Geometry check sheet. Reference: the model listing, model coordinates, mm. Round coordinates to 2 decimals unless told otherwise and drop trailing zeros. Order: outer loops, then holes, each group sorted by start corner. A loop starts at its lowest first (then second) coordinate and runs counter-clockwise, first axis right, second up.
(1) Cross-section at B-B on y = 24.5. Enter the section's corners in (x, z).
(2) Thickness scan on L1, parallel to Y at x = 1.8, z = -2.15; L2, parallel to X at y = -25, z = 1.25; L3, parallel to X at y = -37, z = -1.75. Record the ranges inside material, lowest first.
(3) Gauge pin test, flat ends, axial feed: P1, Ø10, axis at x = -2, y = 32.5, coming from the +Z side; P2, Ø4.5, axis at x = -55, y = 36, coming from the +Z side; P3, Ø2.5, axis at y = 6.5, z = -2, coming from the -X side; P4, Ø1.7, axis at x = 60, y = -36.5, coming from the +Z side. Record the tip position at first contact, or that the pin passes through.
(4) Cross-section at A-A on x = 50.1. Enter the section's corners in (y, z).
(5) Cross-section at C-C on x = 15. Enter the section's corners in (y, z), and give its area (3 significant figures).
Autodesk Inventor part; units mm, degrees
ref_plane "YZ Plane" through (0, 0, 0) normal (1, 0, 0) x (0, 1, 0)
ref_plane "XZ Plane" through (0, 0, 0) normal (0, 1, 0) x (-1, 0, 0)
ref_plane "XY Plane" through (0, 0, 0) normal (0, 0, 1) x (1, 0, 0)
sketch "Sketch1" plane through (0, 0, 0) normal (0, 0, 1) x (1, 0, 0)
  line L0 (65, -35) -> (-65, -35)
  line L1 (-65, -35) -> (-65, 35)
  line L2 (-65, 35) -> (65, 35)
  line L3 (65, 35) -> (65, -35)
  line L4 (65, -35) -> (-65, 35) construction
  line L5 (-65, -35) -> (65, 35) construction
  line L6 (56.8, -15) -> (56.8, -25) construction
  line L7 (54.65, -15) -> (54.65, -25)
  line L8 (58.95, -25) -> (58.95, -15)
  arc A0 (58.95, -15) -> (54.65, -15) centre (56.8, -15) ccw
  arc A1 (54.65, -25) -> (58.95, -25) centre (56.8, -25) ccw
  line L9 (62, -13) -> (65, -13)
  line L10 (65, -13) -> (65, -27)
  line L11 (65, -27) -> (62, -27)
  line L12 (62, -27) -> (62, -13)
  line L13 (62, -13) -> (65, -27) construction
  line L14 (65, -13) -> (62, -27) construction
  line L15 (56.8, -20) -> (63.5, -20) construction
  line L16 (48.6, -13) -> (51.6, -13)
  line L17 (51.6, -13) -> (51.6, -27)
  line L18 (51.6, -27) -> (48.6, -27)
  line L19 (48.6, -27) -> (48.6, -13)
  line L20 (48.6, -13) -> (51.6, -27) construction
  line L21 (51.6, -13) -> (48.6, -27) construction
  line L22 (50.1, -20) -> (56.8, -20) construction
  circle A2 centre (56.8, -20) radius 0.5
  line L23 (56.8, -20) -> (-65, -20)
  line L24 (-60, 35) -> (-60, -35)
  line L25 (-65, 35) -> (65, 35)
  line L26 (65, 35) -> (65, 41)
  line L27 (65, 41) -> (-65, 41)
  line L28 (-65, 41) -> (-65, 35)
  line L29 (-60, 35) -> (-60, 41)
  circle A3 centre (50.1, -13) radius 1.5
  circle A4 centre (63.5, -13) radius 1.5
  circle A5 centre (50.1, -27) radius 1.5
  circle A6 centre (63.5, -27) radius 1.5
  line L30 (-65, -35) -> (-65, -41)
  line L31 (-65, -41) -> (65, -41)
  line L32 (65, -41) -> (65, -35)
  line L33 (-60, -35) -> (-60, -41)
  point P0 (0, 0)
  point P1 (65, -27)
  point P2 (65, -13)
  point P3 (65, -13)
  dimension "d0" = 70
  dimension "d1" = 130
  dimension "d2" = 10
  dimension "d3" = 4.3
  dimension "d4" = 14
  dimension "d5" = 3
  dimension "d6" = 14
  dimension "d7" = 3
  dimension "d10" = 8
  dimension "d11" = 0
  dimension "d16" = 1
  dimension "d20" = 5.2
  dimension "d21" = 5.2
  dimension "d22" = 5
  dimension "d23" = 6
  dimension "d26" = 125
  dimension "d27" = 76
  dimension "d122" = 6
extrude "Extrusion1" add sketch "Sketch1" against normal blind 5 contours L32 L31 L33 L0 | L19 A3 L17 L23 | L23 L17 A5 L19 | L0 L24 L2 L3 A4 L12 A6 | A6 L12 A4 L3 | A6 L11 | L11 A6 | A4 L9 | L9 A4 | L29 L27 L26 L2 | A5 L18 | L18 A5 | A3 L16 | L16 A3
extrude "Extrusion2" add sketch "Sketch1" along normal blind 3 contours L19 A3 L17 L23 | L23 L17 A5 L19 | A6 L12 A4 L3 | A6 L11 | L11 A6 | A4 L9 | L9 A4 | A5 L18 | L18 A5 | A3 L16 | L16 A3
sketch "Sketch4" plane through (0, 0, -5) normal (0, 0, -1) x (-1, 0, 0)
  circle A0 centre (55.4192, -22.54) radius 0.2032 construction
  circle A1 centre (55.4192, -20) radius 0.2032 construction
  circle A2 centre (55.4192, -17.46) radius 0.2032 construction
  circle A3 centre (33.74, 4.2192) radius 0.2032 construction
  circle A4 centre (31.2, 4.2192) radius 0.2032 construction
  circle A5 centre (28.66, 4.2192) radius 0.2032 construction
  circle A6 centre (22.4192, 10.46) radius 0.2032 construction
  circle A7 centre (22.4192, 13) radius 0.2032 construction
  circle A8 centre (22.4192, 15.54) radius 0.2032 construction
  circle A9 centre (-46.0192, 10.46) radius 0.2032 construction
  circle A10 centre (-46.0192, 13) radius 0.2032 construction
  circle A11 centre (-46.0192, 15.54) radius 0.2032 construction
  circle A12 centre (-24.34, 37.2192) radius 0.2032 construction
  circle A13 centre (-21.8, 37.2192) radius 0.2032 construction
  circle A14 centre (-19.26, 37.2192) radius 0.2032 construction
  circle A15 centre (-4.34, 37.2192) radius 0.2032 construction
  circle A16 centre (-1.8, 37.2192) radius 0.2032 construction
  circle A17 centre (0.74, 37.2192) radius 0.2032 construction
  circle A18 centre (55, 36) radius 1.6
  arc A19 (-26.0469, -12.3763) -> (-29.4237, -15.7531) centre (-28.7, -13.1) ccw construction
  arc A20 (-29.4237, -24.2469) -> (-26.0469, -27.6237) centre (-28.7, -26.9) ccw construction
  line L0 (-48.6, -13) -> (-48.6, -27) construction
  circle A21 centre (-56.8, -20) radius 2.3368 construction
  line L1 (-28.7, -26.9) -> (-28.7, -13.1) construction
  line L2 (-56.8, -20) -> (-48.6, -20) construction
  line L3 (-48.6, -20) -> (-28.7, -20) construction
  line L4 (-38.65, -20) -> (-38.65, -36) construction
  line L5 (60, -41) -> (60, 41) construction
  line L6 (60, 36) -> (-65, 36) construction
  line L7 (55, -4) -> (55, 36) construction
  line L8 (-38.65, -20) -> (-38.65, 36) construction
  line L9 (60, 41) -> (-65, 41) construction
  circle A22 centre (-1.8, -4) radius 2.15
  circle A23 centre (14.2, -20) radius 2.15
  line L10 (-1.8, -4) -> (60, -4) construction
  circle A24 centre (55.4192, -22.54) radius 0.5
  circle A25 centre (55.4192, -20) radius 0.5
  circle A26 centre (55.4192, -17.46) radius 0.5
  circle A27 centre (33.74, 4.2192) radius 0.5
  circle A28 centre (31.2, 4.2192) radius 0.5
  circle A29 centre (28.66, 4.2192) radius 0.5
  circle A30 centre (-46.0192, 10.46) radius 0.5
  circle A31 centre (-46.0192, 13) radius 0.5
  circle A32 centre (-46.0192, 15.54) radius 0.5
  circle A33 centre (0.74, 37.2192) radius 0.5
  circle A34 centre (-1.8, 37.2192) radius 0.5
  circle A35 centre (-4.34, 37.2192) radius 0.5
  circle A36 centre (-19.26, 37.2192) radius 0.5
  circle A37 centre (-21.8, 37.2192) radius 0.5
  circle A38 centre (-24.34, 37.2192) radius 0.5
  line L11 (55, -4) -> (55, -35) construction
  line L12 (60, 41) -> (60, -41) construction
  line L13 (60, -36) -> (-65, -36) construction
  circle A39 centre (55, -36) radius 1.6
  line L14 (-60, 41) -> (-60, -35) construction
  circle A40 centre (-60, 36) radius 1.6
  line L15 (22.4192, 13) -> (55, 13) construction
  line L16 (-1.8, -4) -> (-38.65, -4) construction
  circle A41 centre (-38.65, -4) radius 1.6
  line L17 (22.4192, 13) -> (-65, 13) construction
  line L18 (55.4192, -22.54) -> (28.66, -22.54) construction
  line L19 (28.66, -22.54) -> (28.66, 4.2192) construction
  line L20 (28.66, 4.2192) -> (55.4192, 4.2192) construction
  line L21 (55.4192, 4.2192) -> (55.4192, -22.54) construction
  line L22 (-4.34, 37.2192) -> (22.4192, 37.2192) construction
  line L23 (22.4192, 37.2192) -> (22.4192, 10.46) construction
  line L24 (22.4192, 10.46) -> (-4.34, 10.46) construction
  line L25 (-4.34, 10.46) -> (-4.34, 37.2192) construction
  line L26 (-19.26, 37.2192) -> (-46.0192, 37.2192) construction
  line L27 (-46.0192, 37.2192) -> (-46.0192, 10.46) construction
  line L28 (-46.0192, 10.46) -> (-19.26, 10.46) construction
  line L29 (-19.26, 10.46) -> (-19.26, 37.2192) construction
  line L30 (-32.6396, 37.2192) -> (-32.6396, 10.46) construction
  line L31 (-32.6396, 23.8396) -> (-46.0192, 23.8396) construction
  line L32 (-39.3294, 23.8396) -> (-39.3294, 37.2192) construction
  circle A42 centre (-39.3294, 30.5294) radius 1.6
  line L33 (9.0396, 37.2192) -> (9.0396, 10.46) construction
  line L34 (9.0396, 23.8396) -> (22.4192, 23.8396) construction
  line L35 (15.7294, 23.8396) -> (15.7294, 37.2192) construction
  circle A43 centre (15.7294, 30.5294) radius 1.6
  line L36 (42.0396, 4.2192) -> (42.0396, -22.54) construction
  line L37 (42.0396, -9.1604) -> (55.4192, -9.1604) construction
  line L38 (48.7294, -9.1604) -> (48.7294, 4.2192) construction
  circle A44 centre (48.7294, -2.4706) radius 1.6
  circle A45 centre (22.4192, 10.46) radius 0.2032 construction
  circle A46 centre (22.4192, 13) radius 0.2032 construction
  circle A47 centre (22.4192, 15.54) radius 0.2032 construction
  circle A48 centre (22.4192, 15.54) radius 0.5
  circle A49 centre (22.4192, 13) radius 0.5
  circle A50 centre (22.4192, 10.46) radius 0.5
  line L39 (-65, -41) -> (60, -41)
  line L40 (-65, 41) -> (-65, -41)
  circle A51 centre (-60, -36) radius 1.6
  point P0 (0, 0)
  dimension "d29" = 3.2
  dimension "d32" = 5
  dimension "d33" = 5
  dimension "d36" = 1
  dimension "d37" = 1
  dimension "d38" = 1
  dimension "d39" = 1
  dimension "d40" = 1
  dimension "d41" = 1
  dimension "d42" = 1
  dimension "d43" = 1
  dimension "d44" = 1
  dimension "d45" = 1
  dimension "d46" = 1
  dimension "d47" = 1
  dimension "d48" = 1
  dimension "d49" = 1
  dimension "d50" = 1
  dimension "d54" = 3.2
  dimension "d57" = 3.2
  dimension "d59" = 3.2
  dimension "d61" = 3.2
  dimension "d62" = 3.2
  dimension "d63" = 3.2
  dimension "d64" = 1
  dimension "d65" = 1
  dimension "d66" = 1
  dimension "d123" = 5
  dimension "d124" = 5
  dimension "d135" = 3.2
extrude "Extrusion6" cut sketch "Sketch4" against normal up to next
sketch "Sketch7" plane through (0, 0, 0) normal (0, 0, 1) x (1, 0, 0)
  circle A0 centre (-15.7294, 30.5294) radius 1.6
  circle A1 centre (-55.4192, -17.46) radius 0.5
  circle A2 centre (-22.4192, 10.46) radius 0.5
  circle A3 centre (1.8, 37.2192) radius 0.5
  circle A4 centre (24.34, 37.2192) radius 0.5
  circle A5 centre (-14.2, -20) radius 2.15
  circle A6 centre (46.0192, 15.54) radius 0.5
  circle A7 centre (21.8, 37.2192) radius 0.5
  circle A8 centre (-0.74, 37.2192) radius 0.5
  circle A9 centre (-28.66, 4.2192) radius 0.5
  circle A10 centre (-55.4192, -20) radius 0.5
  circle A11 centre (-48.7294, -2.4706) radius 1.6
  circle A12 centre (39.3294, 30.5294) radius 1.6
  circle A13 centre (38.65, -4) radius 1.6
  circle A14 centre (-55, 36) radius 1.6
  circle A15 centre (-33.74, 4.2192) radius 0.5
  circle A16 centre (-22.4192, 13) radius 0.5
  circle A17 centre (4.34, 37.2192) radius 0.5
  circle A18 centre (46.0192, 10.46) radius 0.5
  circle A19 centre (1.8, -4) radius 2.15
  circle A20 centre (46.0192, 13) radius 0.5
  circle A21 centre (19.26, 37.2192) radius 0.5
  circle A22 centre (-22.4192, 15.54) radius 0.5
  circle A23 centre (-31.2, 4.2192) radius 0.5
  circle A24 centre (-55.4192, -22.54) radius 0.5
  circle A25 centre (-55, -36) radius 1.6
  circle A26 centre (60, 36) radius 1.6
  line L0 (54.65, -15) -> (54.65, -25)
  arc A27 (54.65, -25) -> (58.95, -25) centre (56.8, -25) ccw
  line L1 (58.95, -25) -> (58.95, -15)
  arc A28 (58.95, -15) -> (54.65, -15) centre (56.8, -15) ccw
  line L2 (-60, -41) -> (-60, 41)
  line L3 (-60, 41) -> (65, 41)
  circle A29 centre (1.8, -4) radius 4
  circle A30 centre (-14.2, -20) radius 4
  line L4 (52.8, -25) -> (52.8, -15)
  arc A31 (60.8, -15) -> (52.8, -15) centre (56.8, -15) ccw
  line L5 (60.8, -15) -> (60.8, -25)
  arc A32 (52.8, -25) -> (60.8, -25) centre (56.8, -25) ccw
  line L6 (65, 41) -> (65, -41)
  line L7 (65, -41) -> (-60, -41)
  point P0 (0, 0)
  dimension "d69" = 1.85
  dimension "d70" = 1.85
  dimension "d71" = 1.85
sketch "Sketch8" plane through (0, 0, 0) normal (0, 0, 1) x (1, 0, 0)
  circle A0 centre (-48.7294, -2.4706) radius 1.6 construction
  circle A1 centre (-55, 36) radius 1.6 construction
  circle A2 centre (-15.7294, 30.5294) radius 1.6 construction
  circle A3 centre (39.3294, 30.5294) radius 1.6 construction
  circle A4 centre (60, 36) radius 1.6 construction
  circle A5 centre (38.65, -4) radius 1.6 construction
  circle A6 centre (-55, -36) radius 1.6 construction
  circle A7 centre (-55, 36) radius 1.6
  circle A8 centre (-55, 36) radius 2.85
  circle A9 centre (-15.7294, 30.5294) radius 1.6
  circle A10 centre (-15.7294, 30.5294) radius 2.85
  circle A11 centre (39.3294, 30.5294) radius 1.6
  circle A12 centre (39.3294, 30.5294) radius 2.85
  circle A13 centre (60, 36) radius 1.6
  circle A14 centre (60, 36) radius 2.85
  circle A15 centre (-48.7294, -2.4706) radius 2.85
  circle A16 centre (38.65, -4) radius 1.6
  circle A17 centre (38.65, -4) radius 2.85
  circle A18 centre (-55, -36) radius 2.85
  circle A19 centre (60, -36) radius 1.6
  circle A20 centre (60, -36) radius 2.85
  point P0 (0, 0)
  point P1 (0.2167, -2.5455)
  point P2 (0.2167, -5.4545)
  dimension "d72" = 5.7
  dimension "d73" = 5.7
  dimension "d74" = 5.7
  dimension "d75" = 5.7
  dimension "d76" = 5.7
  dimension "d77" = 5.7
  dimension "d78" = 5.7
  dimension "d136" = 5.7
extrude "Extrusion7" cut sketch "Sketch8" against normal blind 2.5 contours A8 | A10 | A12 | A14 | A15 | A16 | A17 | A18 | A20
sketch "Sketch12" plane through (0, 0, 0) normal (0, 0, 1) x (1, 0, 0)
  line L0 (-60, 31.36) -> (-52.8, 31.36)
  line L1 (-52.8, 31.36) -> (-52.8, 20.71)
  line L2 (-52.8, 20.71) -> (-60, 20.71)
  line L3 (-60, 20.71) -> (-60, 31.36)
  line L4 (-58.2, 26.76) -> (-58.2, 26.56) construction
  line L5 (-58.2, 25.51) -> (-58.2, 25.31) construction
  line L6 (-54.75, 21.21) -> (-55.25, 21.21) construction
  line L7 (-54.75, 30.86) -> (-55.25, 30.86) construction
  line L8 (-53.3, 25.586) -> (-53.3, 26.484) construction
  line L9 (-60, 12.432) -> (-52.507, 12.432) construction
  line L10 (-52.507, 12.432) -> (-52.507, 9.9) construction
  line L11 (-52.507, 9.9) -> (-60, 9.9) construction
  line L12 (-60, 0.1) -> (-52.507, 0.1) construction
  line L13 (-52.507, 0.1) -> (-52.507, -2.442) construction
  line L14 (-52.507, -2.442) -> (-60, -2.442) construction
  line L15 (-60, 12.932) -> (-52.007, 12.932)
  line L16 (-52.007, 12.932) -> (-52.007, -2.942)
  line L17 (-52.007, -2.942) -> (-60, -2.942)
  line L18 (-60, -2.942) -> (-60, 12.932)
  line L19 (-60, 41) -> (-60, -41)
  point P0 (0, 0)
  point P1 (-55, 30.86)
  point P2 (-55, 21.21)
  point P3 (-53.3, 26.035)
  point P4 (-58.2, 26.66)
  point P5 (-52.507, 11.166)
  point P6 (-56.2535, 12.432)
  point P7 (-56.2535, -2.442)
  dimension "d148" = 0.5
  dimension "d149" = 0.5
  dimension "d151" = 0.5
  dimension "d152" = 0.5
  dimension "d153" = 0.5
  dimension "d154" = 0
  dimension "d155" = 0
  dimension "d158" = 0.5
extrude "Extrusion12" cut sketch "Sketch12" against normal through all
properties part number "base_main"
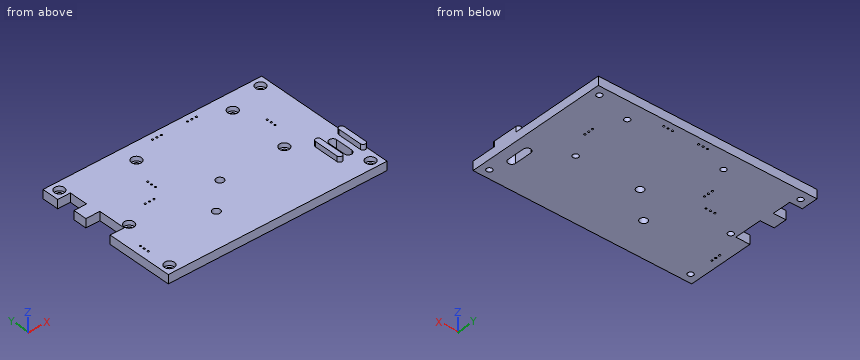
Found:
1. outline: (-52.8, -5) - (65, -5) - (65, 0) - (-52.8, 0) - close
2. L1: y = -41 to -6.15, -1.85 to 36.72, 37.72 to 41
2. L2: x = 48.6 to 51.6, 62 to 65
2. L3: x = -60 to -57.67, -52.33 to 57.33, 62.67 to 65
3. P1: stops at z = 0
3. P2: stops at z = -2.5
3. P3: stops at x = -52.01
3. P4: passes through
4. outline: (-41, -5) - (41, -5) - (41, 0) - (-11.5, 0) - (-11.5, 3) - (-28.5, 3) - (-28.5, 0) - (-41, 0) - close
5. outline: (-41, -5) - (41, -5) - (41, 0) - (-41, 0) - close
5. area: 410 mm2
